Read the model definition and answer for the solid it produces. Units are mm, in the model's axes. A direction names the side the tool comes from. Round coordinates to 2 decimals unless told otherwise and drop trailing zeros. Order: outer loops, then holes, each group sorted by start corner. A loop starts at its lowest first (then second) coordinate and runs counter-clockwise, first axis right, second up. Notation, with made-up numbers: (66.25, 2.25) -> (124.25, 2.25) arc R18 ccw to (124.25, 17.25) -> close; hole circle Ø2 at (12.25, 3). An arc over 180 degrees is marked (long way). Answer as a JSON object with one key per item and string values. Group by question number.
Item 1: Consider probe 1 along X at (y, z) = (-1.5, 1.25); probe 2 along X at (y, z) = (0.75, 6.5). Determine where each line is inside the solid, lowest interval first. Write a range as from..to.
Item 2: Section C-C, the plane z = 8 is taken. Write down the section's boundary in (x, y), plus the area to 3 significant figures.
Item 3: For faces 1 (the flat face through (-0.75, 7, 2)), 2 (the flat face through (-3, -3, 4)), 3 (the flat face through (9, 0, 5)), 4 (the flat face through (0.75, -7, 2)), 5 (the flat face through (0, 9, 5)), determine the directions among +Z, -Z, +X, -X, +Y, -Y from which every point of the face is accessible in a straight line to the end or side of a thin tool.
Item 4: Given P1, Ø2.5, axis at x = -3.5, y = -3.5, coming from the -Z side; P2, Ø1.5, axis at y = 8.5, z = 2.5, coming from the -X side; P3, Ø4, axis at y = -5.5, z = 4, coming from the +X side; P4, Ø1, axis at x = -9.5, z = 6, coming from the +Y side, each flat-ended and moving along its own axis, determine where each tip first touches the part or whether it passes through.
Item 5: Section D-D, the plane y = 8.25 is taken. Write down the section's boundary in (x, z), plus the area to 3 significant figures.
Item 6: Section A-A, the plane x = 0 is taken. Write down the section's boundary in (y, z).
from build123d import *

# Parameters (mm, degrees)
PAD_DEPTH    = 5
SKETCH001_R  = 6
PAD001_DEPTH = 1
SKETCH002_R  = 6
PAD002_DEPTH = 11


with BuildPart() as part:
    # Sketch → Pad (new body)
    with BuildSketch(Plane.XY):
        Polygon((-0.75, 12.5), (-0.75, 0.75), (-12.5, 0.75), (-12.5, -0.75), (-0.75, -0.75), (-0.75, -12.5), (0.75, -12.5), (0.75, -0.75), (12.5, -0.75), (12.5, 0.75), (0.75, 0.75), (0.75, 12.5), align=None)
    extrude(amount=PAD_DEPTH)

    # Sketch001 (on Face14 of Pad) → Pad001 (join)
    with BuildSketch(Plane.XY.offset(5)):
        Circle(SKETCH001_R)
    extrude(amount=-PAD001_DEPTH)

    # Sketch002 (on Face19 of Pad001) → Pad002 (join)
    with BuildSketch(Plane.XY.offset(5)):
        Circle(SKETCH002_R)
    extrude(amount=PAD002_DEPTH)


solid = part.part
Values found:
{
 "1": {"probe 1": "-0.75..0.75", "probe 2": "-5.95..5.95"},
 "2": {"outline": "circle Ø12 at (0, 0)", "area": "113 mm2"},
 "3": {"face 1": "-Z, -X, +Y", "face 2": "-Z, -X, -Y", "face 3": "+Z, +X, +Y, -Y", "face 4": "-Z, +X, -Y", "face 5": "+Z, +X, -X, +Y"},
 "4": {"P1": "z = 4", "P2": "x = -0.75", "P3": "x = 4.87", "P4": "through"},
 "5": {"outline": "(-0.75, 0) -> (0.75, 0) -> (0.75, 5) -> (-0.75, 5) -> close", "area": "7.50 mm2"},
 "6": {"outline": "(-12.5, 0) -> (12.5, 0) -> (12.5, 5) -> (6, 5) -> (6, 16) -> (-6, 16) -> (-6, 5) -> (-12.5, 5) -> close"}
}
